Work out the finished part from the listing and answer in its coordinate system (mm). Face numbers are marked on the shaded views. Coordinates: 2 decimals unless noted, no trailing zeros. Order: outer loops, then holes, each group sorted by start corner. A loop starts at its lowest first (then second) coordinate and runs counter-clockwise, first axis right, second up. Notation, with made-up numbers: (-38.75, -17.5) -> (-7.75, -17.5) arc R24 cw to (-7.75, 14.5) -> close; hole circle Ø9 at (-15, -4). An arc over 180 degrees is marked (long way). Write item = value, one per line. Start each with the question number.
Q1. For a pull along X with two mould halves and no side action, classify the marked faces 1, 2, 3 and 4 as +X half, -X half, draft (parallel to the pull), parting line (faces both ways), or undercut.
Q2. Flat-ended cylindrical pins translate along their axes: pin 1 (6 mm diameter, centred on x = 4.5, z = -2.5, fed in from -Y); pin 2 (2 mm diameter, centred on y = 1.5, z = -8, fed in from -X); pin 3 (0.6 mm diameter, centred on y = -1, z = 2, fed in from -X). Find the tip coordinate at first contact, or state that the pin passes through.
Q3. The part is cut by section C-C, the plane y = 2.05. Determine the outline of the cut face in (x, z), plus the area to 3 significant figures.
Q4. Straight lines are drawn through the part: L1, parallel to Z at x = 1.5, y = 0.55; L2, parallel to Y at x = 0, z = 9.25; L3, parallel to Z at x = 7.25, y = -1.65. For each, find the intervals that lie inside material, in ascending order. Write a range as from..to.
Q5. The part is cut by section A-A, the plane y = 0. Determine the outline of the cut face in (x, z), plus the area to 3 significant figures.
Q6. The part is cut by section D-D, the plane x = 4.75. Determine the outline of the cut face in (y, z).
```python
from build123d import *
from OCP.BRepFilletAPI import BRepFilletAPI_MakeChamfer

# Parameters (mm, degrees)
SKETCH1_R           = 1.190625
EXTRUDE1_DEPTH      = 12.7
SKETCH1_W           = 9.8552
SKETCH1_H           = 1.27
EXTRUDE1_2_DEPTH    = 12.7
SKETCH20_R          = 1.4224
EXTRUDE24_DEPTH     = 20.045522232
CHAMFER2_SIZE       = 0.635
CHAMFER2_SIZE2      = 0.551997079
EXTRUDE4_DEPTH      = 19.94700397
EXTRUDE4_DEPTH_BACK = 19.94700397
SKETCH8_W           = 5.6896
SKETCH8_H           = 8.466666666
SKETCH9_R           = 1.190625
EXTRUDE5_DEPTH      = 8.466666667


# Read off the part's stored shape, not the designer's step: Mirror2
with BuildPart() as part:
    # Sketch1 → Extrude1 (new, symmetric)
    with BuildSketch(Plane.XY):
        with BuildLine():
            Line((12.7, -2.157017049), (1.190625, -2.157017049))
            ThreePointArc((1.190625, -2.157017049), (-1.856577095, 1.619701185), (2.298588957, -0.887017049))
            Line((2.298588957, -0.887017049), (12.7, -0.887017049))
            Line((12.7, -0.887017049), (12.7, -2.157017049))
        make_face()
        Circle(SKETCH1_R, mode=Mode.SUBTRACT)
    extrude(amount=EXTRUDE1_DEPTH, both=True)

    # Mirror2 outline → Mirror2 (revolve, cut)
    with BuildSketch(Plane(origin=(8.3312, 0, -7.8486), x_dir=(1, 0, 0), z_dir=(0, 0, 1))):
        Polygon((1.784715731, -0.887017049), (0, -0.887017049), (0, -1.93881362), (1.4224, -1.93881362), (1.4224, -1.30381362), align=None)
    revolve(axis=Axis((8.3312, 0, -7.8486), (0, 1, 0)), mode=Mode.SUBTRACT)

    # Mirror2 2 outline → Mirror2 2 (revolve, cut)
    with BuildSketch(Plane(origin=(8.3312, 0, 7.8486), x_dir=(1, 0, 0), z_dir=(0, 0, 1))):
        Polygon((0, -0.887017049), (0, -1.93881362), (1.4224, -1.93881362), (1.4224, -1.30381362), (1.784715731, -0.887017049), align=None)
    revolve(axis=Axis((8.3312, 0, 7.8486), (0, 1, 0)), mode=Mode.SUBTRACT)

    # Sketch8 → Extrude4 (cut, two sides: drawn at the far end of the back side and taken through both)
    with BuildSketch(Plane(origin=(0, 0, 0), x_dir=(1, 0, 0), z_dir=(0, 1, 0)).offset(-EXTRUDE4_DEPTH_BACK)):
        Rectangle(SKETCH8_W, SKETCH8_H)
    extrude(amount=EXTRUDE4_DEPTH + EXTRUDE4_DEPTH_BACK, mode=Mode.SUBTRACT)


with BuildPart() as body_2:
    # Sketch1 → Extrude1 2 (new, symmetric)
    with BuildSketch(Plane.XY):
        with Locations((-7.7724, -1.30381362)):
            Rectangle(SKETCH1_W, SKETCH1_H)
    extrude(amount=EXTRUDE1_2_DEPTH, both=True)

    # Sketch20 → Extrude24 (cut, through all)
    with BuildSketch(Plane(origin=(0, -0.66881362, 0), x_dir=(1, 0, 0), z_dir=(0, 1, 0))):
        with Locations(Location((-8.3312, 7.8486, 0), (0, 0, 270))):
            Circle(SKETCH20_R)
        with Locations(Location((-8.3312, -7.8486, 0), (0, 0, 270))):
            Circle(SKETCH20_R)
    extrude(amount=-EXTRUDE24_DEPTH, mode=Mode.SUBTRACT)

    # Chamfer2: one chamfer whose edges measure the first distance from different faces: ONE call of the kernel's chamfer builder (chamfer() names one face for all edges)
    chamfer2_edges_1 = [body_2.edges().sort_by_distance(p)[0] for p in [
        (-8.3312, -0.66881362, -9.271),
    ]]
    chamfer2_side_1 = [body_2.faces().sort_by_distance(p)[0] for p in [
        (-8.3312, -1.30381362, -9.271),
    ]]
    chamfer2_edges_2 = [body_2.edges().sort_by_distance(p)[0] for p in [
        (-8.3312, -0.66881362, 6.4262),
    ]]
    chamfer2_side_2 = [body_2.faces().sort_by_distance(p)[0] for p in [
        (-8.3312, -1.30381362, 6.4262),
    ]]
    chamfer2 = BRepFilletAPI_MakeChamfer(body_2.part.solid().wrapped)
    for e in chamfer2_edges_1:
        chamfer2.Add(CHAMFER2_SIZE, CHAMFER2_SIZE2, e.wrapped, chamfer2_side_1[0].wrapped)  # the first distance lies on this face
    for e in chamfer2_edges_2:
        chamfer2.Add(CHAMFER2_SIZE, CHAMFER2_SIZE2, e.wrapped, chamfer2_side_2[0].wrapped)  # the first distance lies on this face
    add(Compound.cast(chamfer2.Shape()), mode=Mode.REPLACE)

    # Sketch9 → Extrude5 (add)
    with BuildSketch(Plane.XY.offset(-4.233333333)):
        with BuildLine():
            Line((-2.371286314, -0.66881362), (-2.8448, -0.66881362))
            Line((-2.8448, -0.66881362), (-2.8448, -1.93881362))
            Line((-2.8448, -1.93881362), (-1.520300032, -1.93881362))
            ThreePointArc((-1.520300032, -1.93881362), (2.046786768, 1.371486189), (-2.371286314, -0.66881362))
        make_face()
        with Locations(Location((0, 0, 0), (0, 0, 180))):
            Circle(SKETCH9_R, mode=Mode.SUBTRACT)
    extrude(amount=EXTRUDE5_DEPTH)


with BuildPart() as body_3:
    # Sketch6 → Revolve1 (revolve)
    with BuildSketch(Plane(origin=(0, 0, 0), x_dir=(1, 0, 0), z_dir=(0, 1, 0))):
        with BuildLine():
            Line((-2.4638, -12.7), (-2.4638, -13.2715))
            ThreePointArc((-2.4638, -13.2715), (-1.264606924, -13.698253184), (0, -13.843))
            Line((0, -13.843), (0, 13.843))
            ThreePointArc((0, 13.843), (-1.264606924, 13.698253184), (-2.4638, 13.2715))
            Line((-2.4638, 13.2715), (-2.4638, 12.7))
            Line((-2.4638, 12.7), (-1.190625, 12.7))
            Line((-1.190625, 12.7), (-1.190625, -12.7))
            Line((-1.190625, -12.7), (-2.4638, -12.7))
        make_face()
    revolve(axis=Axis((0, 0, -13.843), (0, 0, 1)))


solid = part.part
```
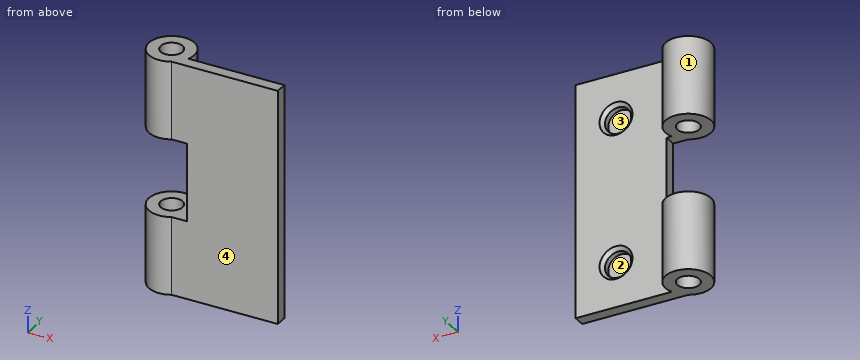
Model answer:
q1.face_1 = parting line
q1.face_2 = undercut
q1.face_3 = undercut
q1.face_4 = draft
q2.pin_1 = -2.16
q2.pin_2 = -2.41
q2.pin_3 = 2.84
q3.outline = (-1.37, -12.7) -> (1.37, -12.7) -> (1.37, -4.23) -> (-1.37, -4.23) -> close; (-1.37, 4.23) -> (1.37, 4.23) -> (1.37, 12.7) -> (-1.37, 12.7) -> close
q3.area = 46.3 mm2
q4.L1 = -12.7..-4.23, 4.23..12.7
q4.L2 = -2.46..-1.19, 1.19..2.46
q4.L3 = -12.7..-8.77, -6.92..6.92, 8.77..12.7
q5.outline = (-2.46, -12.7) -> (-1.19, -12.7) -> (-1.19, -4.23) -> (-2.46, -4.23) -> close; (-2.46, 4.23) -> (-1.19, 4.23) -> (-1.19, 12.7) -> (-2.46, 12.7) -> close; (1.19, -12.7) -> (2.46, -12.7) -> (2.46, -4.23) -> (1.19, -4.23) -> close; (1.19, 4.23) -> (2.46, 4.23) -> (2.46, 12.7) -> (1.19, 12.7) -> close
q5.area = 43.1 mm2
q6.outline = (-2.16, -12.7) -> (-0.89, -12.7) -> (-0.89, 12.7) -> (-2.16, 12.7) -> close
